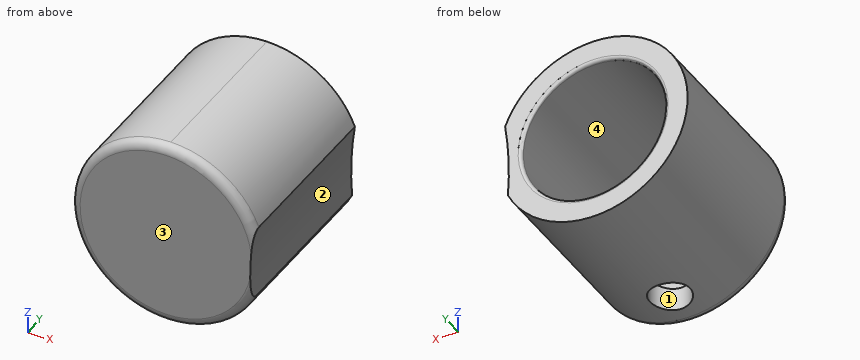
from build123d import *

# Parameters (mm, degrees)
FILLET1_R          = 1.3
SKETCH3_R          = 3
CUT_EXTRUDE1_DEPTH = 20
FILLET3_R          = 0.5
FILLET4_R          = 0.5
CAVITY1_OUTLINE_W  = 50.8
CAVITY1_OUTLINE_H  = 26.650011625


# Read off the part's stored shape, not the designer's step: Cavity1
with BuildPart() as part:
    # Sketch2 → Revolve1 (revolve)
    with BuildSketch(Plane(origin=(0, 0, 0), x_dir=(0, 0, -1), z_dir=(1, 0, 0)), mode=Mode.PRIVATE) as revolve1_sk:
        Polygon((0, 0), (14.115, 0), (14.115, 26.65), (10.7, 26.65), (10.7, 2.79), (0, 2.79), align=None)
    revolve(revolve1_sk.sketch.rotate(Axis((0, 29.213224894, 0), (0, -1, 0)), 180), axis=Axis((0, 29.213224894, 0), (0, -1, 0)))

    # Fillet1
    fillet1_edges = [part.edges().sort_by_distance(p)[0] for p in [
        (0, 0, -14.115),
    ]]
    fillet(fillet1_edges, radius=FILLET1_R)

    # Sketch3 → Cut-Extrude1 (cut)
    with BuildSketch(Plane.XY):
        with Locations((0, 6.37)):
            Circle(SKETCH3_R)
    extrude(amount=-CUT_EXTRUDE1_DEPTH, mode=Mode.SUBTRACT)

    # Fillet3
    fillet3_edges = [part.edges().sort_by_distance(p)[0] for p in [
        (0, 2.79, -10.7),
    ]]
    fillet(fillet3_edges, radius=FILLET3_R)

    # Fillet4
    fillet4_edges = [part.edges().sort_by_distance(p)[0] for p in [
        (0, 26.65, -10.7),
    ]]
    fillet(fillet4_edges, radius=FILLET4_R)

    # Cavity1 outline → Cavity1 (revolve, cut)
    with BuildSketch(Plane(origin=(63.391344809, 0, -2.353004111), x_dir=(1, 0, 0), z_dir=(0, 0, 1))):
        with Locations((25.4, 13.324994188)):
            Rectangle(CAVITY1_OUTLINE_W, CAVITY1_OUTLINE_H)
    revolve(axis=Axis((63.391344809, 0, -2.353004111), (0, 1, 0)), mode=Mode.SUBTRACT)


solid = part.part
Read the model definition and answer for the solid it produces. Units are mm, in the model's axes. Face numbers are marked on the shaded views. Coordinates: 2 decimals unless noted, no trailing zeros. Loops run counter-clockwise (first coordinate to the right, second up) from the corner with the lowest first, then second, coordinate; pieces in that order, holes last.
Q1. The part is cut by section D-D on y = 6.75. Write down the section's boundary in (x, z) (3 decimals).
Q2. The part is cut by section A-A on z = 0. Write down the section's boundary in (x, y) (3 decimals), and give its area (3 significant figures).
Q3. Consider probe 1 along Y at (x, z) = (6, -6); probe 2 along X at (y, z) = (16, 2.5); probe 3 along Z at (x, y) = (-9.5, 14.5). Determine where each line is inside the solid, lowest interval first.
Q4. The mould has two halves that part along X. Classify the marked faces 1, 2, 3 and 4: +X half, -X half, draft (parallel to the pull), parting line (faces both ways), or undercut.
Q5. The part is cut by section B-B on y = 11.75. Write down the section's boundary in (x, z) (3 decimals), and give its area (3 significant figures).
Q6. Each of these flat-tipped pins is pushed along its axis until it touches: pin 1 Ø1.5 at (x, z) = (0, 2.5) entering from +Y; pin 2 Ø6 at (x, y) = (-5, 15.5) entering from -Z; pin 3 Ø2 at (y, z) = (12, -9) entering from +X. Where does it stop, or does it pass through?
Q7. The part is cut by section C-C on y = 4. Write down the section's boundary in (x, z) (3 decimals), and give its area (3 significant figures).
Results below:
1. outline: (-2.976, -13.798) - (-2.976, -10.278) arc R10.7 cw (long way) to (2.976, -10.278) - (2.976, -13.798) arc R14.115 ccw to (12.73, -6.098) arc R50.8 cw to (13.147, 5.138) arc R14.115 ccw (long way) to start
2. outline: (-14.115, 1.3) arc R1.3 ccw to (-12.815, 0) - (12.646, 0) - (12.646, 26.65) - (11.2, 26.65) arc R0.5 ccw to (10.7, 26.15) - (10.7, 3.29) arc R0.5 cw to (10.2, 2.79) - (-10.2, 2.79) arc R0.5 cw to (-10.7, 3.29) - (-10.7, 26.15) arc R0.5 ccw to (-11.2, 26.65) - (-14.115, 26.65) - close
2. area: 202 mm2
3. probe 1: y = 0 to 2.79
3. probe 2: x = -13.89 to -10.4, 10.4 to 12.82
3. probe 3: z = -10.44 to -4.92, 4.92 to 10.44
4. face 1: undercut
4. face 2: +X half
4. face 3: draft
4. face 4: undercut
5. outline: (12.73, -6.098) arc R50.8 cw to (13.147, 5.138) arc R14.115 ccw (long way) to start; hole circle Ø21.4 at (0, 0)
5. area: 255 mm2
6. pin 1: stops at y = 2.79
6. pin 2: stops at z = -13.97
6. pin 3: stops at x = 11.63
7. outline: (-1.839, -13.995) - (-1.839, -10.541) arc R10.7 cw (long way) to (1.839, -10.541) - (1.839, -13.995) arc R14.115 ccw to (12.73, -6.098) arc R50.8 cw to (13.147, 5.138) arc R14.115 ccw (long way) to start
7. area: 242 mm2
